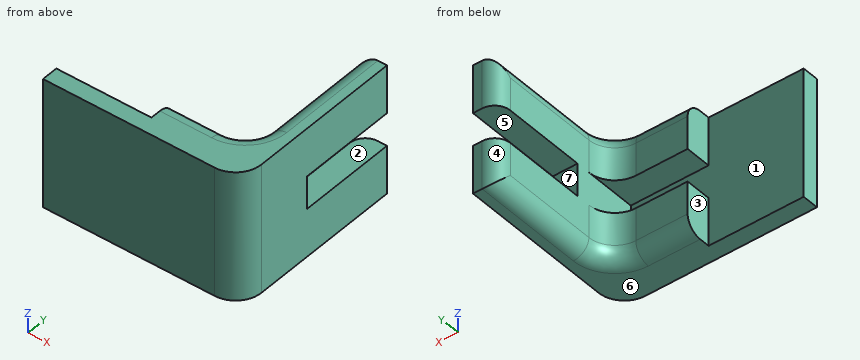
```python
from build123d import *

# Parameters (mm, degrees)
SKETCH1_W           = 76.2
SKETCH1_H           = 50
BOSS_EXTRUDE1_DEPTH = 6.35
SKETCH2_W           = 9.525
SKETCH2_H           = 50
BOSS_EXTRUDE2_DEPTH = 63.5
SKETCH3_W           = 12.7
SKETCH3_H           = 38.1
CUT_EXTRUDE1_DEPTH  = 63.5
SKETCH4_W           = 30
SKETCH4_H           = 50
BOSS_EXTRUDE3_DEPTH = 10
SKETCH5_W           = 30
SKETCH5_H           = 12.7
CUT_EXTRUDE2_DEPTH  = 10
FILLET2_R           = 10
FILLET3_R           = 6
FILLET4_R           = 10


with BuildPart() as part:
    # Sketch1 → Boss-Extrude1 (new body)
    with BuildSketch(Plane(origin=(0, 0, 0), x_dir=(1, 0, 0), z_dir=(0, 1, 0))):
        with Locations((-17.435704212, -13.54987632)):
            Rectangle(SKETCH1_W, SKETCH1_H)
    extrude(amount=BOSS_EXTRUDE1_DEPTH)

    # Sketch2 → Boss-Extrude2 (add)
    with BuildSketch(Plane(origin=(0, 6.35, 0), x_dir=(1, 0, 0), z_dir=(0, 1, 0))):
        with Locations((15.901795788, -13.54987632)):
            Rectangle(SKETCH2_W, SKETCH2_H)
    extrude(amount=BOSS_EXTRUDE2_DEPTH)

    # Sketch3 → Cut-Extrude1 (cut)
    with BuildSketch(Plane.ZY.offset(-11.139295788)):
        with Locations((13.54987632, 50.8)):
            Rectangle(SKETCH3_W, SKETCH3_H)
    extrude(amount=-CUT_EXTRUDE1_DEPTH, mode=Mode.SUBTRACT)

    # Sketch4 → Boss-Extrude3 (add)
    with BuildSketch(Plane(origin=(0, 6.35, 0), x_dir=(1, 0, 0), z_dir=(0, 1, 0))):
        with Locations((-3.860704212, -13.54987632)):
            Rectangle(SKETCH4_W, SKETCH4_H)
    extrude(amount=BOSS_EXTRUDE3_DEPTH)

    # Sketch5 → Cut-Extrude2 (cut)
    with BuildSketch(Plane(origin=(0, 16.35, 0), x_dir=(1, 0, 0), z_dir=(0, 1, 0))):
        with Locations((-3.860704212, -13.54987632)):
            Rectangle(SKETCH5_W, SKETCH5_H)
    extrude(amount=-CUT_EXTRUDE2_DEPTH, mode=Mode.SUBTRACT)

    # Fillet2
    fillet2_edges = [part.edges().sort_by_distance(p)[0] for p in [
        (11.139295788, 16.35, 29.22487632),
        (11.139295788, 16.35, -2.12512368),
    ]]
    fillet(fillet2_edges, radius=FILLET2_R)

    # Fillet3
    fillet3_edges = [part.edges().sort_by_distance(p)[0] for p in [
        (11.139295788, 48.1, -11.45012368),
        (11.139295788, 48.1, 38.54987632),
        (11.139295788, 69.85, -2.12512368),
        (11.139295788, 69.85, 29.22487632),
        (-8.860704212, 16.35, 38.54987632),
        (-8.860704212, 16.35, -11.45012368),
        (8.210363599, 19.278932188, -11.45012368),
        (8.210363599, 19.278932188, 38.54987632),
    ]]
    fillet(fillet3_edges, radius=FILLET3_R)

    # Fillet4
    fillet4_edges = [part.edges().sort_by_distance(p)[0] for p in [
        (20.664295788, 0, 13.54987632),
    ]]
    fillet(fillet4_edges, radius=FILLET4_R)


solid = part.part
```
Geometry: final body of the model. Coordinates: model frame, mm. Face numbers are marked on the shaded views. A direction names the side the tool comes from. Round coordinates to 2 decimals unless told otherwise and drop trailing zeros. Loops run counter-clockwise (first coordinate to the right, second up) from the corner with the lowest first, then second, coordinate; pieces in that order, holes last.
Item 1: Reachability of the marked faces 1, 2 and 3 from +Z, -Z, +X, -X, +Y, -Y: full face, straight path, thin tool, end or side. Return the list, or none.
Checked values:
face 1: -X, +Y
face 2: +X, -X, +Y
face 3: +Z, -Z, -X, +Y
Item 2: Line query: L1, parallel to Y at x = -21, z = 29.5; L2, parallel to X at y = 10, z = -3; L3, parallel to Z at x = 17.5, y = 51. Output: solid intervals per line, ascending.
Checked values:
L1: y = 0 to 6.35
L2: x = -18.86 to 20.66
L3: z = -11.45 to 7.2, 19.9 to 38.55
Item 3: Section C-C, the plane z = 16. Output: boundary loops of the cut face in (x, y).
Checked values:
outline: (-55.54, 0) - (10.66, 0) arc R10 ccw to (20.66, 10) - (20.66, 31.75) - (11.14, 31.75) - (11.14, 6.35) - (-55.54, 6.35) - close
Item 4: Section B-B, the plane x = -1. Output: boundary loops of the cut face in (y, z), plus the area to 3 significant figures.
Checked values:
outline: (0, -11.45) - (10.35, -11.45) arc R6 ccw to (16.35, -5.45) - (16.35, 7.2) - (6.35, 7.2) - (6.35, 19.9) - (16.35, 19.9) - (16.35, 32.55) arc R6 ccw to (10.35, 38.55) - (0, 38.55) - close
area: 675 mm2
Item 5: Mould query, pull axis Z, two halves, no side actions, for the marked faces 4, 5, 6 and 7. Classes: released by +Z, released by -Z, zero draft, split by the parting line, or undercut.
Checked values:
face 4: zero draft
face 5: undercut
face 6: released by -Z
face 7: undercut
Item 6: Contact query for flat-ended pins moving along their axis: P1, Ø3, axis at y = 22, z = 19.5, coming from the -X side; P2, Ø10, axis at x = -13.5, z = -1.5, coming from the +Y side; P3, Ø5, axis at y = 13, z = 32.5, coming from the -X side. Output: stop coordinate, or through.
Checked values:
P1: stops at x = 9.29
P2: stops at y = 16.35
P3: stops at x = -18.86
Item 7: Section A-A, the plane y = 61. Output: boundary loops of the cut face in (x, z).
Checked values:
outline: (11.14, -5.45) arc R6 ccw to (17.14, -11.45) - (20.66, -11.45) - (20.66, 7.2) - (11.14, 7.2) - close; (11.14, 19.9) - (20.66, 19.9) - (20.66, 38.55) - (17.14, 38.55) arc R6 ccw to (11.14, 32.55) - close
Item 8: Section D-D, the plane z = 25. Output: boundary loops of the cut face in (x, y).
Checked values:
outline: (-55.54, 0) - (10.66, 0) arc R10 ccw to (20.66, 10) - (20.66, 69.85) - (17.14, 69.85) arc R6 ccw to (11.14, 63.85) - (11.14, 26.35) arc R10 cw to (1.14, 16.35) - (-18.86, 16.35) - (-18.86, 6.35) - (-55.54, 6.35) - close
